Could you check a few things on this model? Use its own coordinates, in mm. A direction names the side the tool comes from. Round coordinates to 2 decimals unless told otherwise and drop trailing zeros. Order: outer loops, then holes, each group sorted by start corner. A loop starts at its lowest first (then second) coordinate and runs counter-clockwise, first axis right, second up.
```python
from build123d import *

# Parameters (mm, degrees)
SKETCH_1_R          = 3
SKETCH_1_R_2        = 1.5
EXTRUDE_1_DEPTH     = 4
SKETCH_3_R          = 13
CUT_EXTRUDE_2_DEPTH = 2
FILLET_1_R          = 10


with BuildPart() as part:
    # 草图1 → 凸台-拉伸1 (new body)
    with BuildSketch(Plane.XY):
        with BuildLine():
            Line((1791.975111059, 1614.383538533), (1791.975111059, 1566.628704537))
            ThreePointArc((1791.975111059, 1566.628704537), (1790.596787079, 1564.202595154), (1789.871515189, 1561.508200154))
            Line((1789.871515189, 1561.508200154), (1789.871515189, 1513.753366158))
            ThreePointArc((1789.871515189, 1513.753366158), (1793.527688188, 1498.037586639), (1809.60815907, 1499.368670076))
            Line((1809.60815907, 1499.368670076), (1860.094660389, 1562.753352309))
            Line((1860.094660389, 1562.753352309), (1807.257102758, 1618.471746967))
            ThreePointArc((1807.257102758, 1618.471746967), (1798.436490976, 1620.837124602), (1791.975111059, 1614.383538533))
        make_face()
        with Locations((1800.797367784, 1560.012011993)):
            Circle(SKETCH_1_R, mode=Mode.SUBTRACT)
        with Locations((1800.797367784, 1612.012011993)):
            Circle(SKETCH_1_R_2, mode=Mode.SUBTRACT)
        with Locations((1852.797367784, 1560.012011993)):
            Circle(SKETCH_1_R_2, mode=Mode.SUBTRACT)
        with Locations((1800.797367784, 1508.012011993)):
            Circle(SKETCH_1_R_2, mode=Mode.SUBTRACT)
        with BuildLine():
            ThreePointArc((1805.443255224, 1552.809308797), (1806.858027956, 1553.951351821), (1808.000070981, 1555.366124554))
            ThreePointArc((1808.000070981, 1555.366124554), (1807.55260939, 1557.43971519), (1805.479018754, 1556.992253599))
            ThreePointArc((1805.479018754, 1556.992253599), (1804.736707613, 1556.072672165), (1803.817126178, 1555.330361023))
            ThreePointArc((1803.817126178, 1555.330361023), (1803.369664588, 1553.256770387), (1805.443255224, 1552.809308797))
        make_face(mode=Mode.SUBTRACT)
        with BuildLine():
            ThreePointArc((1808.000070981, 1564.657899433), (1806.858027956, 1566.072672165), (1805.443255224, 1567.21471519))
            ThreePointArc((1805.443255224, 1567.21471519), (1803.369664588, 1566.767253599), (1803.817126178, 1564.693662963))
            ThreePointArc((1803.817126178, 1564.693662963), (1804.736707613, 1563.951351821), (1805.479018754, 1563.031770387))
            ThreePointArc((1805.479018754, 1563.031770387), (1807.55260939, 1562.584308797), (1808.000070981, 1564.657899433))
        make_face(mode=Mode.SUBTRACT)
        with BuildLine():
            ThreePointArc((1796.151480345, 1567.21471519), (1794.736707613, 1566.072672165), (1793.594664588, 1564.657899433))
            ThreePointArc((1793.594664588, 1564.657899433), (1794.042126178, 1562.584308797), (1796.115716814, 1563.031770387))
            ThreePointArc((1796.115716814, 1563.031770387), (1796.858027956, 1563.951351821), (1797.77760939, 1564.693662963))
            ThreePointArc((1797.77760939, 1564.693662963), (1798.225070981, 1566.767253599), (1796.151480345, 1567.21471519))
        make_face(mode=Mode.SUBTRACT)
        with BuildLine():
            ThreePointArc((1793.594664588, 1555.366124554), (1794.736707613, 1553.951351821), (1796.151480345, 1552.809308797))
            ThreePointArc((1796.151480345, 1552.809308797), (1798.225070981, 1553.256770387), (1797.77760939, 1555.330361023))
            ThreePointArc((1797.77760939, 1555.330361023), (1796.858027956, 1556.072672165), (1796.115716814, 1556.992253599))
            ThreePointArc((1796.115716814, 1556.992253599), (1794.042126178, 1557.43971519), (1793.594664588, 1555.366124554))
        make_face(mode=Mode.SUBTRACT)
    extrude(amount=EXTRUDE_1_DEPTH)

    # 草图3 → 切除-拉伸2 (cut)
    with BuildSketch(Plane(origin=(0, 0, 0), x_dir=(-1, 0, 0), z_dir=(0, 0, -1))):
        with Locations((-1800.797367784, 1560.012011993)):
            Circle(SKETCH_3_R)
    extrude(amount=-CUT_EXTRUDE_2_DEPTH, mode=Mode.SUBTRACT)

    # 圆角1
    fillet_1_edges = [part.edges().sort_by_distance(p)[0] for p in [
        (1860.094660389, 1562.753352309, 2),
    ]]
    fillet(fillet_1_edges, radius=FILLET_1_R)


solid = part.part
```
Q1. Imagine slicing it at B-B, the plane x = 1832. Please give me the cut outline in (y, z), then the cut area to 3 significant figures.
Q2. I need wall thicknesses on L1, parallel to Y at x = 1807.5, z = 2.25; L2, parallel to X at y = 1566, z = 3.55; L3, parallel to Y at x = 1800.5, z = 1. Which ranges of each line are inside material? Lowest first, please.
Q3. Imagine slicing it at C-C, the plane y = 1580. Please give me the cut outline in (x, z).
Q4. Imagine slicing it at A-A, the plane z = 3.35. State how many separate pieces and enclosed holes the cut face has, then the cut area to 3 significant figures.
Q5. For P1, Ø1.8, axis at x = 1800.8, y = 1508.01, coming from the +Z side; P2, Ø2, axis at y = 1594.5, z = 2.5, coming from the -X side; P3, Ø2, axis at y = 1538.5, z = 1.5, coming from the -X side, each with a flat end and sliding along its axis, tell me the tip position at first contact or that it passes through.
Q6. For faces 1 (the flat face through (1805, 1560, 2)), 2 (the cylindrical face through (1794.755, 1566.091, 2.986)), 3 (the flat face through (1791.975, 1591, 2)), which set-ups out of +Z, -Z, +X, -X, +Y, -Y let a thin tool reach every point of the face, with its end or its side?
Filled in:
1. outline: (1527.48, 0) - (1592.38, 0) - (1592.38, 4) - (1527.48, 4) - close
1. area: 260 mm2
2. L1: y = 1497.65 to 1554.67, 1557.47 to 1562.55, 1565.35 to 1618.22
2. L2: x = 1791.54 to 1794.66, 1798.46 to 1803.13, 1806.93 to 1856.1
2. L3: y = 1495.67 to 1506.54, 1509.48 to 1547.02, 1573.01 to 1610.54, 1613.48 to 1621.14
3. outline: (1791.98, 0) - (1843.74, 0) - (1843.74, 4) - (1791.98, 4) - close
4. separate pieces: 1
4. enclosed holes: 8
4. area: 5,120 mm2
5. P1: passes through
5. P2: stops at x = 1791.98
5. P3: stops at x = 1789.87
6. face 1: -Z
6. face 2: +Z, -Z
6. face 3: +Z, -Z, -X, +Y
